Can you work these out from the model? Positions are in its coordinate system, mm. Face numbers are marked on the shaded views. A direction names the side the tool comes from. Coordinates: 2 decimals unless noted, no trailing zeros. Order: outer loops, then holes, each group sorted by start corner. A loop starts at its lowest first (then second) coordinate and runs counter-clockwise, first axis right, second up. Notation, with made-up numbers: (33, 63.5) -> (80, 63.5) arc R35 ccw to (80, 100.5) -> close; hole circle Ø9 at (0.25, 32). An arc over 180 degrees is marked (long way). Use a Markdown table: item, result. Add a question column.
1. For the marked faces 1 and 2, which set-ups out of +Z, -Z, +X, -X, +Y, -Y let a thin tool reach every point of the face, with its end or its side?
2. We'd pull the mould along Y, two halves only. Please class the marked faces 3, 4 and 5: pulls with the +Y half, pulls with the -Y half, needs draft (parallel to the pull), parting line crosses it, or undercut.
3. Suppose I cut it at B-B, the plane x = 9.25. List the corners of the cut face in (y, z) for me, then the cut area to 3 significant figures.
4. If I drill on line 1 along Z through (x, y) = (5.5, 8.5); line 2 along X through (y, z) = (7.75, -12.25); line 3 along Z through (x, y) = (5.25, 11.5), over which ranges is the centre line in solid material (lowest first)? Write a range as from..to.
5. For pin 1 Ø5 at (x, y) = (5, 8) entering from +Z; pin 2 Ø1 at (x, z) = (9.5, -13) entering from -Y; pin 3 Ø1.5 at (x, z) = (6.5, -13) entering from -Y; pin 4 Ø1 at (x, y) = (5, 2) entering from +Z, each with a flat end and sliding along its axis, tell me the tip position at first contact or that it passes through.
6. Suppose I cut it at A-A, the plane y = 6.75. List the corners of the cut face in (x, z) for me, then the cut area to 3 significant figures.
7. Suppose I cut it at D-D, the plane x = 6.5. List the corners of the cut face in (y, z) for me.
8. Suppose I cut it at C-C, the plane z = -12.55. List the corners of the cut face in (x, y) for me, then the cut area to 3 significant figures.
```python
from build123d import *

# Parameters (mm, degrees)
BOX_W        = 10
BOX_H        = 12
BOX_DEPTH    = 2
SKETCH_R     = 4.25
PAD_DEPTH    = 2
SKETCH001_R  = 2
POCKET_DEPTH = 1


with BuildPart() as part:
    # Box → Box (new body)
    with BuildSketch(Plane.XY):
        with Locations((5, 6)):
            Rectangle(BOX_W, BOX_H)
    extrude(amount=BOX_DEPTH)

    # Sketch → Pad (new body)
    with BuildSketch(Plane.XY.offset(2)):
        with Locations((4.904306, 7.272724)):
            Circle(SKETCH_R)
    extrude(amount=PAD_DEPTH)

    # Sketch001 → Pocket (cut)
    with BuildSketch(Plane.XY.offset(4)):
        with Locations((4.904306, 7.272724)):
            Circle(SKETCH001_R)
    extrude(amount=-POCKET_DEPTH, mode=Mode.SUBTRACT)


with BuildPart() as part_1:
    # Clone placement: moved
    add(part.part.moved(Location((1.5, 0, -16))))


solid = part_1.part
```
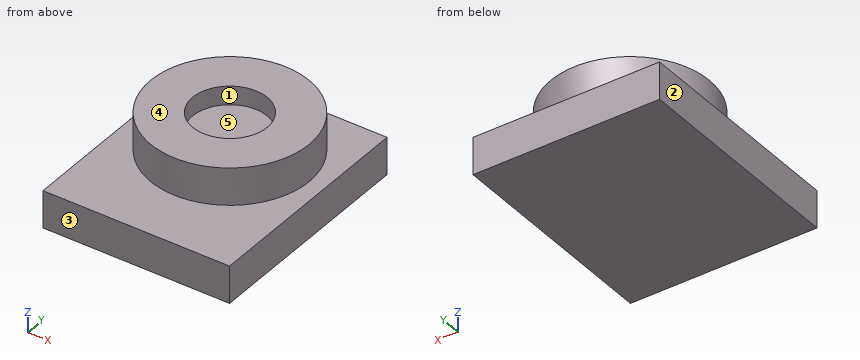
Worked out:
| question | item | result |
|---|---|---|
| 1 | face 1 | +Z |
| 1 | face 2 | +Z, -Z, -X, +Y, -Y |
| 2 | face 3 | pulls with the -Y half |
| 2 | face 4 | needs draft |
| 2 | face 5 | undercut |
| 3 | outline | (0, -16) -> (12, -16) -> (12, -14) -> (10.43, -14) -> (10.43, -12) -> (4.12, -12) -> (4.12, -14) -> (0, -14) -> close |
| 3 | area | 36.6 mm² |
| 4 | line 1 | z = -16..-13 |
| 4 | line 2 | x = 2.18..4.46, 8.35..10.63 |
| 4 | line 3 | z = -16..-14 |
| 5 | pin 1 | stops at z = -12 |
| 5 | pin 2 | stops at y = 3.91 |
| 5 | pin 3 | stops at y = 3.02 |
| 5 | pin 4 | stops at z = -14 |
| 6 | outline | (1.5, -16) -> (11.5, -16) -> (11.5, -14) -> (10.62, -14) -> (10.62, -12) -> (8.33, -12) -> (8.33, -13) -> (4.47, -13) -> (4.47, -12) -> (2.19, -12) -> (2.19, -14) -> (1.5, -14) -> close |
| 6 | area | 33.0 mm² |
| 7 | outline | (0, -16) -> (12, -16) -> (12, -14) -> (11.52, -14) -> (11.52, -12) -> (9.27, -12) -> (9.27, -13) -> (5.28, -13) -> (5.28, -12) -> (3.02, -12) -> (3.02, -14) -> (0, -14) -> close |
| 8 | outline | circle Ø8.5 at (6.4, 7.27); hole circle Ø4 at (6.4, 7.27) |
| 8 | area | 44.2 mm² |
